Geometry check sheet. Reference: the model listing, model coordinates, mm. Face numbers are marked on the shaded views. A direction names the side the tool comes from. Round coordinates to 2 decimals unless told otherwise and drop trailing zeros. Order: outer loops, then holes, each group sorted by start corner. A loop starts at its lowest first (then second) coordinate and runs counter-clockwise, first axis right, second up. Notation, with made-up numbers: (86, -31.75) -> (90, -31.75) arc R6 ccw to (90, -24.75) -> close; hole circle Ø9 at (38.25, -16.5). An arc over 180 degrees is marked (long way). Use a Markdown table: item, result. Add a question column.
Item 1: Sectioned sample at C-C, the plane x = -24.5. Record the cut outline in (y, z).
Item 2: Sectioned sample at A-A, the plane y = 38.75. Record the cut outline in (x, z), and give its area (3 significant figures).
Item 3: Set-up check for the marked faces 1 and 2: record each of +Z, -Z, +X, -X, +Y, -Y from which the full face is reachable in a straight line by a thin tool's end or side.
Item 4: Sectioned sample at D-D, the plane z = 70.5. Record the cut outline in (x, y), and give its area (3 significant figures).
Item 5: Gauge pin test, flat end, axial feed: pin 1 Ø4 at (x, y) = (-63.5, 37) entering from -Z. Record the tip position at first contact, or that the pin passes through.
Item 6: Material ranges on probe 1 along X at (y, z) = (55.5, 170.5); probe 2 along Y at (x, z) = (-52, 155.5); probe 3 along X at (y, z) = (58, 190.5), recorded low to high. Write a range as [from, to].
Item 7: Sectioned sample at B-B, the plane z = 241.3. State how many separate pieces and enclosed holes the cut face has, and give its area (3 significant figures).
from build123d import *

# Parameters (mm, degrees)
F0_W     = 50.8
F0_H     = 25.4
F1_DEPTH = 254
F3_D     = 5.1054
F4_W     = 47.5996
F4_H     = 22.225
F5_DEPTH = 254
F7_D     = 5.1054


with BuildPart() as f1:
    # F0 (on Top) → F1 (new body)
    with BuildSketch(Plane.XY):
        with Locations((-43.475499, 46.040844)):
            Rectangle(F0_W, F0_H)
    extrude(amount=F1_DEPTH)

    # F3 (through all)
    with Locations(Plane.XZ.offset(-33.340844)):
        with Locations((-56.175499, 165.1), (-56.175499, 88.9), (-56.175499, 139.7), (-56.175499, 114.3), (-30.775499, 165.1), (-30.775499, 114.3), (-30.775499, 12.7), (-30.775499, 63.5), (-56.175499, 38.1), (-56.175499, 63.5), (-30.775499, 38.1), (-30.775499, 88.9), (-56.175499, 12.7), (-30.775499, 139.7), (-30.775499, 215.9), (-30.775499, 190.5), (-30.775499, 241.3), (-56.175499, 241.3), (-56.175499, 215.9), (-56.175499, 190.5)):
            Hole(F3_D / 2)

    # F4 (on face) → F5 (cut)
    with BuildSketch(Plane.XY.offset(254)):
        with Locations((-43.475499, 46.040844)):
            Rectangle(F4_W, F4_H)
    extrude(amount=-F5_DEPTH, mode=Mode.SUBTRACT)

    # F7 (through all)
    with Locations(Plane(origin=(-68.875499, 0, 0), x_dir=(0, -1, 0), z_dir=(-1, 0, 0))):
        with Locations((-46.040844, 241.3), (-46.040844, 139.7), (-46.040844, 165.1), (-46.040844, 88.9), (-46.040844, 114.3), (-46.040844, 63.5), (-46.040844, 190.5), (-46.040844, 215.9), (-46.040844, 38.1), (-20.640844, 241.3), (-46.040844, 12.7)):
            Hole(F7_D / 2)


solid = f1.part
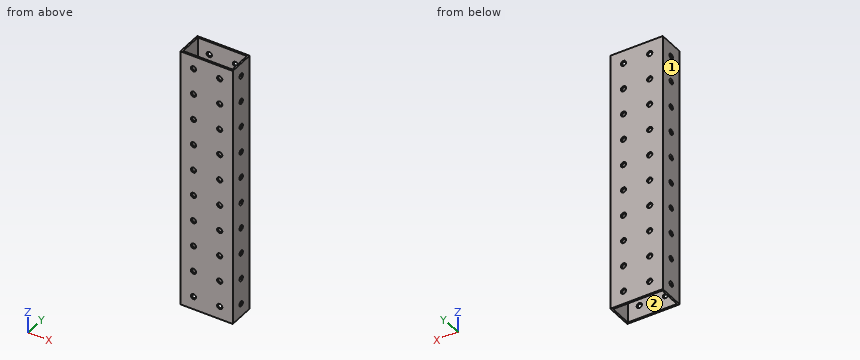
Found:
| question | item | result |
|---|---|---|
| 1 | outline | (33.34, 0) -> (34.93, 0) -> (34.93, 254) -> (33.34, 254) -> close; (57.15, 0) -> (58.74, 0) -> (58.74, 254) -> (57.15, 254) -> close |
| 2 | outline | (-68.88, 0) -> (-67.28, 0) -> (-67.28, 254) -> (-68.88, 254) -> close; (-19.68, 0) -> (-18.08, 0) -> (-18.08, 254) -> (-19.68, 254) -> close |
| 2 | area | 813 mm2 |
| 3 | face 1 | +Z, -Z, -X, +Y, -Y |
| 3 | face 2 | +Z, -Z |
| 4 | outline | (-68.88, 33.34) -> (-18.08, 33.34) -> (-18.08, 58.74) -> (-68.88, 58.74) -> close; hole (-67.28, 34.93) -> (-19.68, 34.93) -> (-19.68, 57.15) -> (-67.28, 57.15) -> close |
| 4 | area | 232 mm2 |
| 5 | pin 1 | passes through |
| 6 | probe 1 | x = [-68.88, -67.28], [-19.68, -18.08] |
| 6 | probe 2 | y = [33.34, 34.93], [57.15, 58.74] |
| 6 | probe 3 | x = [-68.88, -58.73], [-53.62, -33.33], [-28.22, -18.08] |
| 7 | separate pieces | 6 |
| 7 | enclosed holes | 0 |
| 7 | area | 184 mm2 |
